from build123d import *

# Parameters (mm, degrees)
SKETCH1_R           = 35
BOSS_EXTRUDE2_DEPTH = 3.25


with BuildPart() as part:
    # Sketch1 → Boss-Extrude2 (new body)
    # profile 1 of 18: a face of its own
    with BuildSketch(Plane.XY):
        with BuildLine():
            ThreePointArc((-22.640281254, -46.997360821), (4.870724861, -54.696758811), (32.381730977, -46.997360821))
            ThreePointArc((32.381730977, -46.997360821), (38.582870536, -42.59286173), (44.089679783, -37.346072617))
            ThreePointArc((44.089679783, -37.346072617), (54.305553731, -20.806905189), (57.870724861, -1.696758811))
            ThreePointArc((57.870724861, -1.696758811), (54.305553731, 17.413387567), (44.089679783, 33.952554996))
            ThreePointArc((44.089679783, 33.952554996), (37.500783054, 40.067811131), (29.973177775, 44.981575111))
            ThreePointArc((29.973177775, 44.981575111), (22.997792458, 48.106950091), (15.645384984, 50.19646521))
            ThreePointArc((15.645384984, 50.19646521), (4.870724861, 51.303241189), (-5.903935262, 50.19646521))
            ThreePointArc((-5.903935262, 50.19646521), (-13.256342735, 48.106950091), (-20.231728052, 44.981575111))
            ThreePointArc((-20.231728052, 44.981575111), (-27.759333331, 40.067811131), (-34.34823006, 33.952554996))
            ThreePointArc((-34.34823006, 33.952554996), (-48.129275139, -1.696758811), (-34.34823006, -37.346072617))
            ThreePointArc((-34.34823006, -37.346072617), (-28.841420813, -42.59286173), (-22.640281254, -46.997360821))
        make_face()
        with BuildLine():
            ThreePointArc((54.820105173, -1.696758811), (53.54559302, -12.908261975), (49.787097659, -23.547618021))
            ThreePointArc((49.787097659, -23.547618021), (46.308922772, -29.586117847), (42.024200497, -35.081783024))
            ThreePointArc((42.024200497, -35.081783024), (36.642437794, -40.238928584), (30.553154788, -44.537783385))
            ThreePointArc((30.553154788, -44.537783385), (24.340896907, -47.695160892), (17.749674274, -49.957231825))
            ThreePointArc((17.749674274, -49.957231825), (4.870724861, -51.646139122), (-8.008224552, -49.957231825))
            ThreePointArc((-8.008224552, -49.957231825), (-14.599447184, -47.695160892), (-20.811705065, -44.537783385))
            ThreePointArc((-20.811705065, -44.537783385), (-26.900988071, -40.238928584), (-32.282750775, -35.081783024))
            ThreePointArc((-32.282750775, -35.081783024), (-36.567473049, -29.586117847), (-40.045647936, -23.547618021))
            ThreePointArc((-40.045647936, -23.547618021), (-45.07865545, -1.696758811), (-40.045647936, 20.1541004))
            ThreePointArc((-40.045647936, 20.1541004), (-36.567473049, 26.192600226), (-32.282750775, 31.688265402))
            ThreePointArc((-32.282750775, 31.688265402), (-25.881184313, 37.663890011), (-18.5343822, 42.429668157))
            ThreePointArc((-18.5343822, 42.429668157), (-12.212969352, 45.240305281), (-5.563843448, 47.150558185))
            ThreePointArc((-5.563843448, 47.150558185), (4.870724861, 48.252621501), (15.305293171, 47.150558185))
            Line((15.305293171, 47.150558185), (15.315817601, 47.200071738))
            ThreePointArc((15.315817601, 47.200071738), (21.971732028, 45.287872229), (28.299596439, 42.474362712))
            Line((28.299596439, 42.474362712), (28.275831923, 42.429668157))
            ThreePointArc((28.275831923, 42.429668157), (35.622634036, 37.663890011), (42.024200497, 31.688265402))
            ThreePointArc((42.024200497, 31.688265402), (46.308922772, 26.192600226), (49.787097659, 20.1541004))
            ThreePointArc((49.787097659, 20.1541004), (53.54559302, 9.514744354), (54.820105173, -1.696758811))
        make_face(mode=Mode.SUBTRACT)
    # profile 2 of 18: a face of its own
    with BuildSketch(Plane.XY):
        with BuildLine():
            Line((-17.374636259, 40.248503273), (-18.5343822, 42.429668157))
            ThreePointArc((-18.5343822, 42.429668157), (-25.881184313, 37.663890011), (-32.282750775, 31.688265402))
            Line((-32.282750775, 31.688265402), (-30.446943745, 30.035297329))
            Line((-30.446943745, 30.035297329), (-26.772022731, 30.227891778))
            ThreePointArc((-26.772022731, 30.227891778), (-22.802876936, 33.723836243), (-18.450553688, 36.729335933))
            Line((-18.450553688, 36.729335933), (-17.374636259, 40.248503273))
        make_face()
    # profile 3 of 18: a face of its own
    with BuildSketch(Plane.XY):
        with BuildLine():
            Line((-13.288474299, 28.223860933), (-18.450553688, 36.729335933))
            ThreePointArc((-18.450553688, 36.729335933), (-22.802876936, 33.723836243), (-26.772022731, 30.227891778))
            Line((-26.772022731, 30.227891778), (-19.76801672, 23.161487574))
            ThreePointArc((-19.76801672, 23.161487574), (-16.677426775, 25.883617566), (-13.288474299, 28.223860933))
        make_face()
    # profile 4 of 18: a face of its own
    with BuildSketch(Plane.XY):
        with Locations((4.870724861, -1.696758811)):
            Circle(SKETCH1_R)
    # profile 5 of 18: a face of its own
    with BuildSketch(Plane.XY):
        with BuildLine():
            ThreePointArc((-34.345862627, 20.26926168), (-40.07865545, -1.696758811), (-34.345862627, -23.662779301))
            Line((-34.345862627, -23.662779301), (-25.66541496, -18.800681308))
            ThreePointArc((-25.66541496, -18.800681308), (-30.128946569, -1.84841548), (-25.812491143, 15.141894807))
            Line((-25.812491143, 15.141894807), (-34.345862627, 20.26926168))
        make_face()
    # profile 6 of 18: a face of its own
    with BuildSketch(Plane.XY):
        with BuildLine():
            ThreePointArc((-40.045647936, 20.1541004), (-45.07865545, -1.696758811), (-40.045647936, -23.547618021))
            Line((-40.045647936, -23.547618021), (-37.825337209, -22.464700122))
            Line((-37.825337209, -22.464700122), (-34.345862627, -23.662779301))
            ThreePointArc((-34.345862627, -23.662779301), (-40.07865545, -1.696758811), (-34.345862627, 20.26926168))
            Line((-34.345862627, 20.26926168), (-37.825337209, 19.071182501))
            Line((-37.825337209, 19.071182501), (-40.045647936, 20.1541004))
        make_face()
    # profile 7 of 18: a face of its own
    with BuildSketch(Plane.XY):
        with BuildLine():
            ThreePointArc((-32.282750775, -35.081783024), (-26.900988071, -40.238928584), (-20.811705065, -44.537783385))
            Line((-20.811705065, -44.537783385), (-19.539395166, -42.420304124))
            Line((-19.539395166, -42.420304124), (-20.4296591, -38.849650513))
            ThreePointArc((-20.4296591, -38.849650513), (-23.72059697, -36.380805667), (-26.772022731, -33.621409399))
            Line((-26.772022731, -33.621409399), (-30.446943745, -33.42881495))
            Line((-30.446943745, -33.42881495), (-32.282750775, -35.081783024))
        make_face()
    # profile 8 of 18: a face of its own
    with BuildSketch(Plane.XY):
        with BuildLine():
            ThreePointArc((-26.772022731, -33.621409399), (-23.72059697, -36.380805667), (-20.4296591, -38.849650513))
            Line((-20.4296591, -38.849650513), (-14.829511994, -30.625994332))
            ThreePointArc((-14.829511994, -30.625994332), (-17.392012848, -28.703619229), (-19.76801672, -26.555005195))
            Line((-19.76801672, -26.555005195), (-26.772022731, -33.621409399))
        make_face()
    # profile 9 of 18: a face of its own
    with BuildSketch(Plane.XY):
        with BuildLine():
            ThreePointArc((-9.208840303, -44.384141433), (4.870724861, -46.646139122), (18.950290026, -44.384141433))
            Line((18.950290026, -44.384141433), (15.833829966, -34.935446006))
            ThreePointArc((15.833829966, -34.935446006), (4.870724861, -36.696758811), (-6.092380244, -34.935446006))
            Line((-6.092380244, -34.935446006), (-9.208840303, -44.384141433))
        make_face()
    # profile 10 of 18: a face of its own
    with BuildSketch(Plane.XY):
        with BuildLine():
            ThreePointArc((-8.008224552, -49.957231825), (4.870724861, -51.646139122), (17.749674274, -49.957231825))
            Line((17.749674274, -49.957231825), (17.110307887, -47.571083983))
            Line((17.110307887, -47.571083983), (18.950290026, -44.384141433))
            ThreePointArc((18.950290026, -44.384141433), (4.870724861, -46.646139122), (-9.208840303, -44.384141433))
            Line((-9.208840303, -44.384141433), (-7.368858164, -47.571083983))
            Line((-7.368858164, -47.571083983), (-8.008224552, -49.957231825))
        make_face()
    # profile 11 of 18: a face of its own
    with BuildSketch(Plane.XY):
        with BuildLine():
            Line((14.791684342, 44.734218625), (15.305293171, 47.150558185))
            ThreePointArc((15.305293171, 47.150558185), (4.870724861, 48.252621501), (-5.563843448, 47.150558185))
            Line((-5.563843448, 47.150558185), (-5.05023462, 44.734218625))
            Line((-5.05023462, 44.734218625), (-1.963956889, 42.729966432))
            ThreePointArc((-1.963956889, 42.729966432), (4.870724861, 43.252621501), (11.705406612, 42.729966432))
            Line((11.705406612, 42.729966432), (14.791684342, 44.734218625))
        make_face()
    # profile 12 of 18: a face of its own
    with BuildSketch(Plane.XY):
        with BuildLine():
            Line((10.192574898, 32.896273901), (11.705406612, 42.729966432))
            ThreePointArc((11.705406612, 42.729966432), (4.870724861, 43.252621501), (-1.963956889, 42.729966432))
            Line((-1.963956889, 42.729966432), (-0.451125175, 32.896273901))
            ThreePointArc((-0.451125175, 32.896273901), (4.870724861, 33.303241189), (10.192574898, 32.896273901))
        make_face()
    # profile 13 of 18: a face of its own
    with BuildSketch(Plane.XY):
        with BuildLine():
            Line((40.188393468, 30.035297329), (42.024200497, 31.688265402))
            ThreePointArc((42.024200497, 31.688265402), (35.622634036, 37.663890011), (28.275831923, 42.429668157))
            Line((28.275831923, 42.429668157), (27.116085982, 40.248503273))
            Line((27.116085982, 40.248503273), (28.192003411, 36.729335933))
            ThreePointArc((28.192003411, 36.729335933), (32.544326659, 33.723836243), (36.513472454, 30.227891778))
            Line((36.513472454, 30.227891778), (40.188393468, 30.035297329))
        make_face()
    # profile 14 of 18: a face of its own
    with BuildSketch(Plane.XY):
        with BuildLine():
            Line((29.509466442, 23.161487574), (36.513472454, 30.227891778))
            ThreePointArc((36.513472454, 30.227891778), (32.544326659, 33.723836243), (28.192003411, 36.729335933))
            Line((28.192003411, 36.729335933), (22.897057483, 28.304096714))
            ThreePointArc((22.897057483, 28.304096714), (26.357668487, 25.931329318), (29.509466442, 23.161487574))
        make_face()
    # profile 15 of 18: a face of its own
    with BuildSketch(Plane.XY):
        with BuildLine():
            Line((35.406864683, -18.800681308), (44.08731235, -23.662779301))
            ThreePointArc((44.08731235, -23.662779301), (48.363299492, -13.047650513), (49.820105173, -1.696758811))
            ThreePointArc((49.820105173, -1.696758811), (48.363299492, 9.654132891), (44.08731235, 20.26926168))
            Line((44.08731235, 20.26926168), (35.406864683, 15.407163687))
            ThreePointArc((35.406864683, 15.407163687), (38.736377769, 7.141654685), (39.870724861, -1.696758811))
            ThreePointArc((39.870724861, -1.696758811), (38.736377769, -10.535172306), (35.406864683, -18.800681308))
        make_face()
    # profile 16 of 18: a face of its own
    with BuildSketch(Plane.XY):
        with BuildLine():
            Line((47.566786932, -22.464700122), (49.787097659, -23.547618021))
            ThreePointArc((49.787097659, -23.547618021), (53.54559302, -12.908261975), (54.820105173, -1.696758811))
            ThreePointArc((54.820105173, -1.696758811), (53.54559302, 9.514744354), (49.787097659, 20.1541004))
            Line((49.787097659, 20.1541004), (47.566786932, 19.071182501))
            Line((47.566786932, 19.071182501), (44.08731235, 20.26926168))
            ThreePointArc((44.08731235, 20.26926168), (48.363299492, 9.654132891), (49.820105173, -1.696758811))
            ThreePointArc((49.820105173, -1.696758811), (48.363299492, -13.047650513), (44.08731235, -23.662779301))
            Line((44.08731235, -23.662779301), (47.566786932, -22.464700122))
        make_face()
    # profile 17 of 18: a face of its own
    with BuildSketch(Plane.XY):
        with BuildLine():
            ThreePointArc((30.553154788, -44.537783385), (36.642437794, -40.238928584), (42.024200497, -35.081783024))
            Line((42.024200497, -35.081783024), (40.188393468, -33.42881495))
            Line((40.188393468, -33.42881495), (36.513472454, -33.621409399))
            ThreePointArc((36.513472454, -33.621409399), (33.462046693, -36.380805667), (30.171108822, -38.849650513))
            Line((30.171108822, -38.849650513), (29.280844889, -42.420304124))
            Line((29.280844889, -42.420304124), (30.553154788, -44.537783385))
        make_face()
    # profile 18 of 18: a face of its own
    with BuildSketch(Plane.XY):
        with BuildLine():
            ThreePointArc((30.171108822, -38.849650513), (33.462046693, -36.380805667), (36.513472454, -33.621409399))
            Line((36.513472454, -33.621409399), (29.509466442, -26.555005195))
            ThreePointArc((29.509466442, -26.555005195), (27.133462571, -28.703619229), (24.570961717, -30.625994332))
            Line((24.570961717, -30.625994332), (30.171108822, -38.849650513))
        make_face()
    extrude(amount=BOSS_EXTRUDE2_DEPTH)


solid = part.part
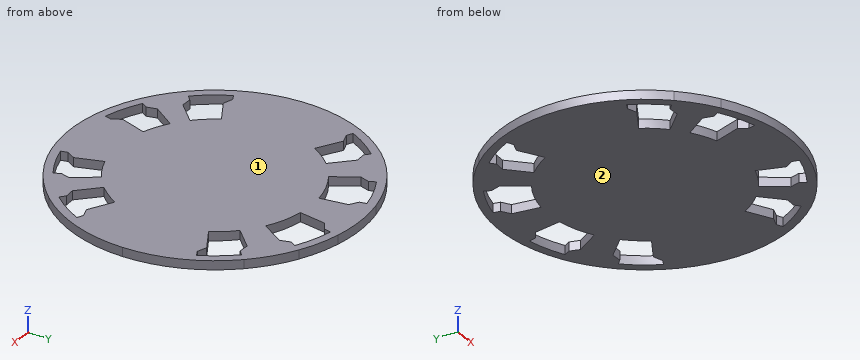
Geometry: final body of the model. Coordinates: model frame, mm. Face numbers are marked on the shaded views. Give positions to 0.01 mm unless a question says otherwise; leave off trailing zeros. Write each loop counter-clockwise with the first axis right and the second up, starting at its lowest first coordinate (ties: lowest second). Pieces come first, ordered by that corner, then holes.
(1) Mould query, pull axis Z, two halves, no side actions, for the marked faces 1 and 2. Classes: released by +Z, released by -Z, zero draft, split by the parting line, or undercut.
(2) First-contact query: P1, Ø1, axis at x = 34, z = 1, coming from the +Y side. Flat tip, straight axial feed; report the tip coordinate or a pass-through.
(3) Ray query, line 1 (Y direction, x = -20.5, z = 3.1); line 2 (X direction, y = -24.5, z = 0.25); line 3 (Y direction, x = 45, z = 1.05) (3 decimals). Return the intervals inside material, ascending.
(4) Cut plane C-C, the plane y = -28.5. Return loops of the section in (x, z).
(5) Cut plane A-A, the plane y = 25. Return loops of the section in (x, z), then the cut area to 3 significant figures.
(6) Cut plane B-B, the plane z = 2.7. Give the number of separate pieces and of enclosed holes in the cut face, then the cut area to 3 significant figures.
Values follow:
1. face 1: released by +Z
1. face 2: released by -Z
2. P1: stops at y = 42.91
3. line 1: y = -48.23 to -44.72, -44.02 to -27.29, -25.81 to 22.41, 23.9 to 44.84
3. line 2: x = -42.97 to -39.57, -21.68 to 31.42, 49.31 to 52.71
3. line 3: y = -36.318 to -31.439, -23.349 to 19.955, 28.045 to 32.925
4. outline: (-40.85, 0) - (-37.28, 0) - (-37.28, 3.25) - (-40.85, 3.25) - close; (-21.7, 0) - (31.44, 0) - (31.44, 3.25) - (-21.7, 3.25) - close; (47.02, 0) - (50.59, 0) - (50.59, 3.25) - (47.02, 3.25) - close
5. outline: (-40.91, 0) - (-37.35, 0) - (-37.35, 3.25) - (-40.91, 3.25) - close; (-21.59, 0) - (31.33, 0) - (31.33, 3.25) - (-21.59, 3.25) - close; (47.09, 0) - (50.66, 0) - (50.66, 3.25) - (47.09, 3.25) - close
5. area: 195 mm2
6. separate pieces: 1
6. enclosed holes: 8
6. area: 7,300 mm2
